from build123d import *

# Parameters (mm, degrees)
F0_W     = 17.5
F0_H     = 15.5
F1_DEPTH = 2
F2_DEPTH = 3
F3_DEPTH = 1


with BuildPart() as f1:
    # F0 (on Top) → F1 (new body)
    with BuildSketch(Plane.XY):
        Polygon((-8.75, -7.75), (-8.75, -9.75), (10.75, -9.75), (10.75, 9.75), (-8.75, 9.75), (-8.75, 7.75), (8.75, 7.75), (8.75, -7.75), align=None)
        Rectangle(F0_W, F0_H)
        Polygon((-10.75, 9.75), (-10.75, -9.75), (-8.75, -9.75), (-8.75, -7.75), (-8.75, 7.75), (-8.75, 9.75), align=None)
    extrude(amount=F1_DEPTH)

    # F0 (on Top) → F2 (join)
    with BuildSketch(Plane.XY):
        Rectangle(F0_W, F0_H)
        Polygon((-8.75, -7.75), (-8.75, -9.75), (10.75, -9.75), (10.75, 9.75), (-8.75, 9.75), (-8.75, 7.75), (8.75, 7.75), (8.75, -7.75), align=None)
    extrude(amount=-F2_DEPTH)

    # F0 (on Top) → F3 (cut)
    with BuildSketch(Plane.XY):
        Polygon((-8.75, -7.75), (-8.75, -9.75), (10.75, -9.75), (10.75, 9.75), (-8.75, 9.75), (-8.75, 7.75), (8.75, 7.75), (8.75, -7.75), align=None)
    extrude(amount=-F3_DEPTH, mode=Mode.SUBTRACT)


solid = f1.part
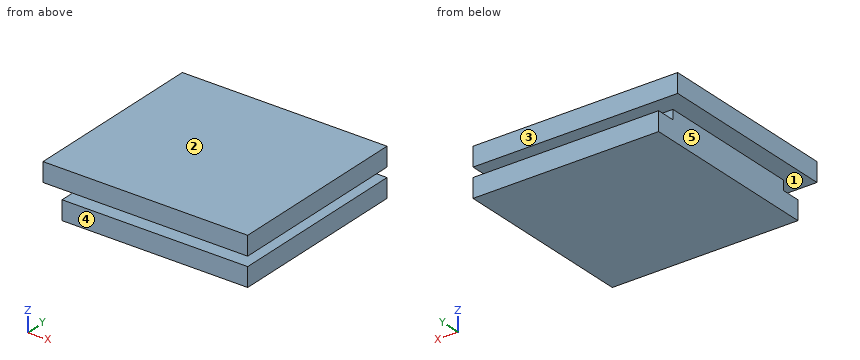
Input: part model. Units: mm. Frame: model coordinates. Face numbers are marked on the shaded views. A direction names the side the tool comes from. Give positions to 0.01 mm unless a question says otherwise; leave off trailing zeros. Write each loop counter-clockwise with the first axis right and the second up, starting at its lowest first coordinate (ties: lowest second). Pieces come first, ordered by that corner, then holes. Notation, with made-up numbers: (11, 74.5) -> (63, 74.5) arc R23 cw to (63, 101.5) -> close; hole circle Ø5 at (31, 43.25). An arc over 180 degrees is marked (long way). Use one line per item in the form item = value. Start each with the question number.
1) Section query D-D on y = -5.75. Return the cut outline in (x, z).
2) Ray query, probe 1 along Z at (x, y) = (-0.5, -8.5); probe 2 along Y at (x, z) = (5.25, -0.15); probe 3 along X at (y, z) = (-1, -0.8). Return the intervals inside material, ascending. Write a range as from..to.
3) Draft query along Z for the marked faces 1, 2 and 3. Return one class per face: pulls with the +Z half, pulls with the -Z half, needs draft (parallel to the pull), parting line crosses it, or undercut.
4) Pin query (flat end, axial travel): pin 1 (0.8 mm diameter, centred on x = 3, z = -0.5, fed in from -Y); pin 2 (1.5 mm diameter, centred on y = -0.5, z = -2, fed in from -X); pin 3 (0.8 mm diameter, centred on y = 2, z = -0.5, fed in from +X). Return the tip coordinate at first contact, or that it passes through.
5) Set-up query: the marked faces 4 and 5. Return all of +Z, -Z, +X, -X, +Y, -Y with unobstructed straight access to the full face (end or side cutting, diameter ignored); none if empty.
6) Section query B-B on x = -2. Return the cut outline in (y, z), then the cut area to 3 significant figures.
7) Section query C-C on z = -0.4. Return the cut outline in (x, y).
8) Section query A-A on y = 8.75. Return the cut outline in (x, z), then the cut area to 3 significant figures.
Outcome:
q1.outline = (-10.75, 0) -> (-8.75, 0) -> (-8.75, -3) -> (10.75, -3) -> (10.75, -1) -> (8.75, -1) -> (8.75, 0) -> (10.75, 0) -> (10.75, 2) -> (-10.75, 2) -> close
q2.probe_1 = -3..-1, 0..2
q2.probe_2 = -7.75..7.75
q2.probe_3 = -8.75..8.75
q3.face_1 = undercut
q3.face_2 = pulls with the +Z half
q3.face_3 = needs draft
q4.pin_1 = -7.75
q4.pin_2 = -8.75
q4.pin_3 = 8.75
q5.face_4 = +Z, -Z, +X, -X, -Y
q5.face_5 = -Z, -X, +Y, -Y
q6.outline = (-9.75, -3) -> (9.75, -3) -> (9.75, -1) -> (7.75, -1) -> (7.75, 0) -> (9.75, 0) -> (9.75, 2) -> (-9.75, 2) -> (-9.75, 0) -> (-7.75, 0) -> (-7.75, -1) -> (-9.75, -1) -> close
q6.area = 93.5 mm^2
q7.outline = (-8.75, -7.75) -> (8.75, -7.75) -> (8.75, 7.75) -> (-8.75, 7.75) -> close
q8.outline = (-10.75, 0) -> (10.75, 0) -> (10.75, 2) -> (-10.75, 2) -> close; (-8.75, -3) -> (10.75, -3) -> (10.75, -1) -> (-8.75, -1) -> close
q8.area = 82.0 mm^2
